Could you check a few things on this model? Use its own coordinates, in mm. Face numbers are marked on the shaded views. A direction names the side the tool comes from. Round coordinates to 2 decimals unless told otherwise and drop trailing zeros. Loops run counter-clockwise (first coordinate to the right, second up) from the corner with the lowest first, then second, coordinate; pieces in that order, holes last. Notation, with made-up numbers: M 26,-4.75 L 74,-4.75 A14 cw 74,19.25 Z; hole C -28,41.25 d10. An arc over 180 degrees is marked long. One line per item, written item: value. Start each with the question number.
Q1. Imagine slicing it at C-C (x = -6). Please give me the cut outline in (y, z).
Q2. Imagine slicing it at B-B (y = 0.5). Please give me the cut outline in (x, z), then the cut area to 3 significant figures.
Q3. I'm going to push flat-ended pins straight in: pin 1 Ø1.5 at (x, y) = (-2, 2) entering from +Z; pin 2 Ø3 at (x, y) = (10, -1) entering from -Z; pin 3 Ø3.5 at (x, z) = (20.29, 5) entering from +Y; pin 4 Ø2.5 at (x, y) = (-2, -1.5) entering from -Z. Where does each tip first touch, or does it pass through?
Q4. Imagine slicing it at A-A (z = 5). Please give me the cut outline in (x, y), then the cut area to 3 significant figures.
Q5. Please list where these lines run through material, in increasing order: line 1 along X through (y, z) = (-2.5, 6); line 2 along Z through (x, y) = (-11, 4); line 3 along Y through (x, z) = (21, 2).
Q6. Thinking about a two-plate mould opening in X: for the marked faces 6, 7 and 8, which applies, released by +X, released by -X, zero draft, split by the parting line, or undercut?
Q7. Which directions (+Z, -Z, +X, -X, +Y, -Y) give clear straight access to the entire face, cutting with the end or side of a thin tool? Please do the marked faces 1, 2, 3, 4 and 5.
Q8. Imagine slicing it at D-D (y = -4.5). Please give me the cut outline in (x, z) (3 decimals), then the cut area to 3 significant figures.
from build123d import *

# Parameters (mm, degrees)
BOSS_EXTRUDE1_DEPTH             = 10
SKETCH2_R                       = 1.925
CUT_EXTRUDE1_DEPTH              = 29.104589728
BOSS_EXTRUDE2_REACH             = 28.737
BOSS_EXTRUDE2_DIRECTION_2_REACH = 28.737
SKETCH4_R                       = 1.925
CUT_EXTRUDE2_DEPTH              = 29.980475562
FILLET1_START                   = -6
FILLET1_DEPTH                   = 12
FILLET1_START_2                 = -5
FILLET1_2_DEPTH                 = 10
FILLET2_R                       = 2


with BuildPart() as part:
    # Sketch1 → Boss-Extrude1 (new body)
    with BuildSketch(Plane.XY):
        with BuildLine():
            Line((-0.712802471, 5), (-0.712802471, 0))
            Line((-0.712802471, 0), (11.232311414, 0))
            ThreePointArc((11.232311414, 0), (13.199986934, 2.636374102), (16.287197529, 1.5))
            Line((16.287197529, 1.5), (24.287197529, 1.5))
            Line((24.287197529, 1.5), (24.287197529, 5))
            Line((24.287197529, 5), (-0.712802471, 5))
        make_face()
        with BuildLine():
            Line((11.232311414, 0), (-0.712802471, 0))
            Line((-0.712802471, 0), (-0.712802471, -5))
            Line((-0.712802471, -5), (24.287197529, -5))
            Line((24.287197529, -5), (24.287197529, -1.5))
            Line((24.287197529, -1.5), (16.287197529, -1.5))
            ThreePointArc((16.287197529, -1.5), (13.199986934, -2.636374102), (11.232311414, 0))
        make_face()
    extrude(amount=BOSS_EXTRUDE1_DEPTH)

    # Sketch2 → Cut-Extrude1 (cut, through all)
    with BuildSketch(Plane(origin=(0, 5, 0), x_dir=(1, 0, 0), z_dir=(0, 1, 0))):
        with Locations(Location((20.287197529, -5, 0), (0, 0, 270))):
            Circle(SKETCH2_R)
    extrude(amount=-CUT_EXTRUDE1_DEPTH, mode=Mode.SUBTRACT)

    # Boss-Extrude2: up to this face of the body (flat: up to its plane)
    boss_extrude2_end = Plane(part.part.faces().sort_by_distance((11.372052598, 5, 5))[0])
    # Sketch3 → Boss-Extrude2 (add, up to the picked face)
    with BuildSketch(Plane(origin=(0, 0, 0), x_dir=(1, 0, 0), z_dir=(0, 1, 0)), mode=Mode.PRIVATE) as boss_extrude2_sk1:
        Polygon((-0.712802471, 0), (-3.712802471, 0), (-3.712802471, 2.5), (-16.712802471, 2.5), (-16.712802471, -0.5), (-6.712802471, -0.5), (-6.712802471, -3), (-0.712802471, -3), align=None)
    boss_extrude2_tool1 = split(extrude(boss_extrude2_sk1.sketch, amount=BOSS_EXTRUDE2_REACH, mode=Mode.PRIVATE), bisect_by=boss_extrude2_end, keep=Keep.BOTH, mode=Mode.PRIVATE)
    # Sketch3 → Boss-Extrude2 (add, up to the picked face)
    with BuildSketch(Plane(origin=(0, 0, 0), x_dir=(1, 0, 0), z_dir=(0, 1, 0)), mode=Mode.PRIVATE) as boss_extrude2_sk2:
        Polygon((-0.712802471, -7), (-6.712802471, -7), (-6.712802471, -9.5), (-16.712802471, -9.5), (-16.712802471, -12.5), (-3.712802471, -12.5), (-3.712802471, -10), (-0.712802471, -10), align=None)
    boss_extrude2_tool2 = split(extrude(boss_extrude2_sk2.sketch, amount=BOSS_EXTRUDE2_REACH, mode=Mode.PRIVATE), bisect_by=boss_extrude2_end, keep=Keep.BOTH, mode=Mode.PRIVATE)
    add(boss_extrude2_tool1.solids().sort_by(Axis((-8.239829, 0, -0.222973), (0, 1, 0)))[0])
    add(boss_extrude2_tool2.solids().sort_by(Axis((-8.239829, 0, 10.222973), (0, 1, 0)))[0])

    # Boss-Extrude2 direction 2: up to this face of the body (flat: up to its plane)
    boss_extrude2_direction_2_end = Plane(part.part.faces().sort_by_distance((11.372052598, -5, 5))[0])
    # Sketch3 → Boss-Extrude2 direction 2 (add, up to the picked face)
    with BuildSketch(Plane(origin=(0, 0, 0), x_dir=(1, 0, 0), z_dir=(0, 1, 0)), mode=Mode.PRIVATE) as boss_extrude2_direction_2_sk1:
        Polygon((-0.712802471, 0), (-3.712802471, 0), (-3.712802471, 2.5), (-16.712802471, 2.5), (-16.712802471, -0.5), (-6.712802471, -0.5), (-6.712802471, -3), (-0.712802471, -3), align=None)
    boss_extrude2_direction_2_tool1 = split(extrude(boss_extrude2_direction_2_sk1.sketch, amount=-BOSS_EXTRUDE2_DIRECTION_2_REACH, mode=Mode.PRIVATE), bisect_by=boss_extrude2_direction_2_end, keep=Keep.BOTH, mode=Mode.PRIVATE)
    # Sketch3 → Boss-Extrude2 direction 2 (add, up to the picked face)
    with BuildSketch(Plane(origin=(0, 0, 0), x_dir=(1, 0, 0), z_dir=(0, 1, 0)), mode=Mode.PRIVATE) as boss_extrude2_direction_2_sk2:
        Polygon((-0.712802471, -7), (-6.712802471, -7), (-6.712802471, -9.5), (-16.712802471, -9.5), (-16.712802471, -12.5), (-3.712802471, -12.5), (-3.712802471, -10), (-0.712802471, -10), align=None)
    boss_extrude2_direction_2_tool2 = split(extrude(boss_extrude2_direction_2_sk2.sketch, amount=-BOSS_EXTRUDE2_DIRECTION_2_REACH, mode=Mode.PRIVATE), bisect_by=boss_extrude2_direction_2_end, keep=Keep.BOTH, mode=Mode.PRIVATE)
    add(boss_extrude2_direction_2_tool1.solids().sort_by(Axis((-8.239829, 0, -0.222973), (0, -1, 0)))[0])
    add(boss_extrude2_direction_2_tool2.solids().sort_by(Axis((-8.239829, 0, 10.222973), (0, -1, 0)))[0])

    # Sketch4 → Cut-Extrude2 (cut, through all)
    with BuildSketch(Plane.XY.offset(12.5)):
        with Locations((-12.212802471, 0)):
            Circle(SKETCH4_R)
    extrude(amount=-CUT_EXTRUDE2_DEPTH, mode=Mode.SUBTRACT)

    # Fillet1: read off the stored shape, not the designer's step
    # Fillet1 outline → Fillet1 (cut)
    with BuildSketch(Plane(origin=(0, 0, 0), x_dir=(1, 0, 0), z_dir=(0, 1, 0)).offset(FILLET1_START)):
        with BuildLine():
            Line((-6.712802471, -7), (-6.712802471, -9.5))
            ThreePointArc((-6.712802471, -9.5), (-5.691254253, -7.708712153), (-3.75476258, -7))
            Line((-3.75476258, -7), (-6.712802471, -7))
        make_face()
        with BuildLine():
            ThreePointArc((-3.75476258, -3), (-5.691254253, -2.291287847), (-6.712802471, -0.5))
            Line((-6.712802471, -0.5), (-6.712802471, -3))
            Line((-6.712802471, -3), (-3.75476258, -3))
        make_face()
    extrude(amount=FILLET1_DEPTH, mode=Mode.SUBTRACT)

    # Fillet1 2 outline → Fillet1 2 (add)
    with BuildSketch(Plane(origin=(0, 0, 0), x_dir=(1, 0, 0), z_dir=(0, 1, 0)).offset(FILLET1_START_2)):
        with BuildLine():
            Line((-3.712802471, -10), (-3.712802471, -12.5))
            ThreePointArc((-3.712802471, -12.5), (-2.691254253, -10.708712153), (-0.75476258, -10))
            Line((-0.75476258, -10), (-3.712802471, -10))
        make_face()
        with BuildLine():
            ThreePointArc((-0.75476258, 0), (-2.691254253, 0.708712153), (-3.712802471, 2.5))
            Line((-3.712802471, 2.5), (-3.712802471, 0))
            Line((-3.712802471, 0), (-0.75476258, 0))
        make_face()
    extrude(amount=FILLET1_2_DEPTH)

    # Fillet2
    fillet2_edges = [part.edges().sort_by_distance(p)[0] for p in [
        (24.287197529, 3.25, 0),
        (24.287197529, -3.25, 0),
        (24.287197529, -3.25, 10),
        (24.287197529, 3.25, 10),
        (-16.712802471, 0, -2.5),
        (-16.712802471, 0, 12.5),
    ]]
    fillet(fillet2_edges, radius=FILLET2_R)


solid = part.part
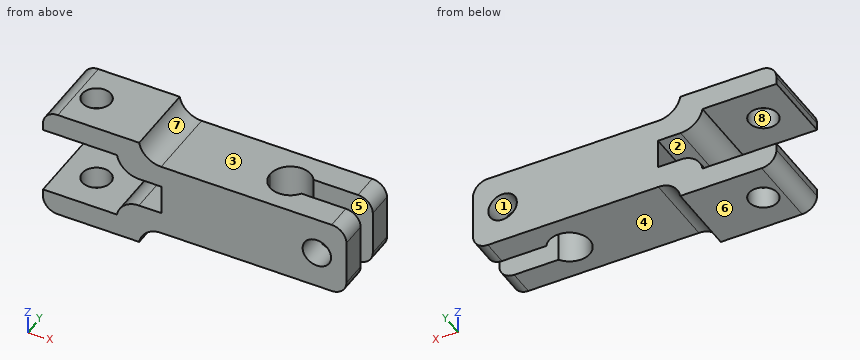
Report:
1. outline: M -5,-2.5 L 5,-2.5 L 5,1.99 L -5,1.99 Z; M -5,8.01 L 5,8.01 L 5,12.5 L -5,12.5 Z
2. outline: M -16.71,-0.5 A2 ccw -14.71,-2.5 L -14.07,-2.5 L -14.07,0.5 L -16.71,0.5 Z; M -16.71,9.5 L -14.07,9.5 L -14.07,12.5 L -14.71,12.5 A2 ccw -16.71,10.5 Z; M -10.35,-2.5 L -3.71,-2.5 A3 cw -0.75,0 L 11.28,0 L 11.28,10 L -0.75,10 A3 cw -3.71,12.5 L -10.35,12.5 L -10.35,9.5 L -6.71,9.5 A3 ccw -3.75,7 L -0.71,7 L -0.71,3 L -3.75,3 A3 ccw -6.71,0.5 L -10.35,0.5 Z
2. area: 207 mm²
3. pin 1: stops at z = 10.76
3. pin 2: stops at z = 0
3. pin 3: passes through
3. pin 4: stops at z = -1.33
4. outline: M -0.71,-5 L 18.36,-5 L 18.36,-1.5 L 16.29,-1.5 A2.75 cw long 16.29,1.5 L 18.36,1.5 L 18.36,5 L -0.71,5 Z; M 22.21,-5 L 24.29,-5 L 24.29,-1.5 L 22.21,-1.5 Z; M 22.21,1.5 L 24.29,1.5 L 24.29,5 L 22.21,5 Z
4. area: 176 mm²
5. line 1: x = -0.71 to 12.84, 15.13 to 18.64, 21.93 to 24.29
5. line 2: z = -2.5 to 0.5, 9.5 to 12.5
5. line 3: y = -5 to -1.5, 1.5 to 5
6. face 6: zero draft
6. face 7: released by +X
6. face 8: undercut
7. face 1: +Y, -Y
7. face 2: -X, +Y, -Y
7. face 3: +Z, +X, +Y, -Y
7. face 4: -Z, +X, +Y, -Y
7. face 5: +Z, -Z, +X
8. outline: M -16.713,-0.5 A2 ccw -14.713,-2.5 L -3.713,-2.5 A3 cw -0.755,0 L 22.287,0 A2 ccw 24.287,2 L 24.287,8 A2 ccw 22.287,10 L -0.755,10 A3 cw -3.713,12.5 L -14.713,12.5 A2 ccw -16.713,10.5 L -16.713,9.5 L -6.713,9.5 A3 ccw -3.755,7 L -0.713,7 L -0.713,3 L -3.755,3 A3 ccw -6.713,0.5 L -16.713,0.5 Z; hole C 20.287,5 d3.85
8. area: 346 mm²
